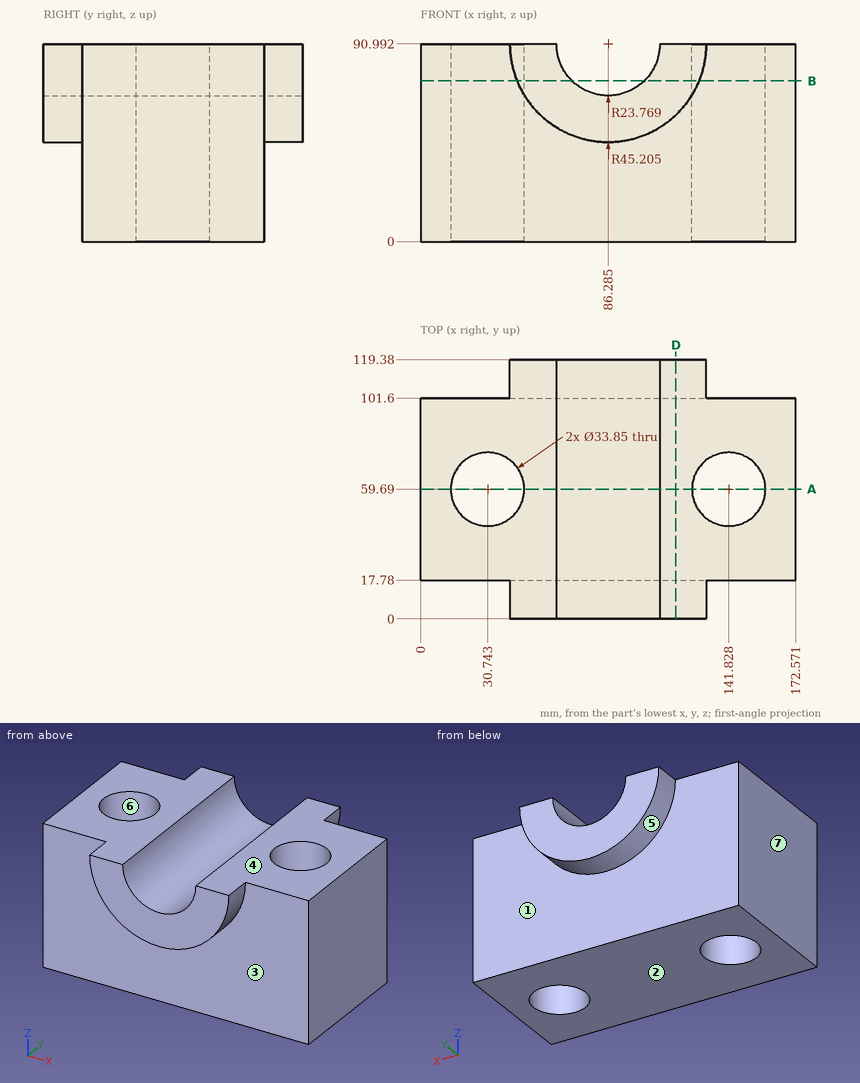
Check sheet for the drawn part. Datum: minimum x, y, z corner. Units: mm. A direction names the side the tool comes from. Coordinates: 2 decimals unless noted, no trailing zeros. Write each loop counter-clockwise with the first axis right and the second up, starting at its lowest first coordinate (ties: lowest second). Pieces come first, ordered by that corner, then holes. Notation, with made-up numbers: M -16.5,-34 L 18.5,-34 A27 cw 18.5,-10 Z; hole C 30.5,29 d10. An arc over 180 degrees is marked long. Use a Markdown table: item, result.
Q1. Sectioned sample at A-A, the plane y = 59.69. Record the boundary of the cut face in (x, z) (1 decimal).
Reply:
| item | result |
|---|---|
| outline | M 0,0 L 13.8,0 L 13.8,91 L 0,91 Z; M 47.7,0 L 124.9,0 L 124.9,91 L 110.1,91 A23.8 cw 62.5,91 L 47.7,91 Z; M 158.8,0 L 172.6,0 L 172.6,91 L 158.8,91 Z |
Q2. Sectioned sample at D-D, the plane x = 117.5. Record the boundary of the cut face in (y, z) (1 decimal), plus the area to 3 significant figures.
Reply:
| item | result |
|---|---|
| outline | M 0,58.3 L 17.8,58.3 L 17.8,0 L 101.6,0 L 101.6,58.3 L 119.4,58.3 L 119.4,91 L 0,91 Z |
| area | 8,790 mm² |
Q3. Draft check along X on the marked faces 4, 5, 6 and 7. Enter one of: +X half, -X half, draft (parallel to the pull), parting line (faces both ways), or undercut.
Reply:
| item | result |
|---|---|
| face 4 | draft |
| face 5 | parting line |
| face 6 | undercut |
| face 7 | -X half |
Q4. Thickness scan on line 1 (X direction, y = 59, z = 60); line 2 (X direction, y = 59.69, z = 27.5); line 3 (Y direction, x = 86, z = 39). Record the ranges inside material, lowest first.
Reply:
| item | result |
|---|---|
| line 1 | x = 0 to 13.83, 47.65 to 124.92, 158.74 to 172.57 |
| line 2 | x = 0 to 13.82, 47.67 to 124.9, 158.75 to 172.57 |
| line 3 | y = 17.78 to 101.6 |
Q5. Set-up check for the marked faces 1, 2 and 3: record each of +Z, -Z, +X, -X, +Y, -Y from which the full face is reachable in a straight line by a thin tool's end or side.
Reply:
| item | result |
|---|---|
| face 1 | -Z, +Y |
| face 2 | -Z, +X, -X, +Y, -Y |
| face 3 | -Z, -Y |
Q6. Go/stop test with flat-tipped pins: P1, Ø10, axis at x = 64, z = 29.5, coming from the -Y side; P2, Ø6, axis at x = 50, z = 11.5, coming from the +Y side. Record where each tip stops, or that it passes through.
Reply:
| item | result |
|---|---|
| P1 | stops at y = 17.78 |
| P2 | stops at y = 101.6 |
Q7. Sectioned sample at B-B, the plane z = 74. Count the separate pieces of the cut face and the enclosed holes in it, plus the area to 3 significant figures.
Reply:
| item | result |
|---|---|
| separate pieces | 2 |
| enclosed holes | 2 |
| area | 11,700 mm² |
